Study the drawing (mm; zero at the part's minimum x, y, z) and answer. Give positions to 0.01 mm unless a question says otherwise; leave off trailing zeros. Order: outer loops, then holes, each group sorted by start corner. A loop starts at its lowest first (then second) coordinate and runs counter-clockwise, first axis right, second up. Notation, with made-up numbers: (39.5, 6.5) - (68.5, 6.5) arc R19 cw to (68.5, 14.5) - close; hole circle Ø11 at (89.25, 9.5). An arc over 180 degrees is marked (long way). Put each result on its own line as item: value.
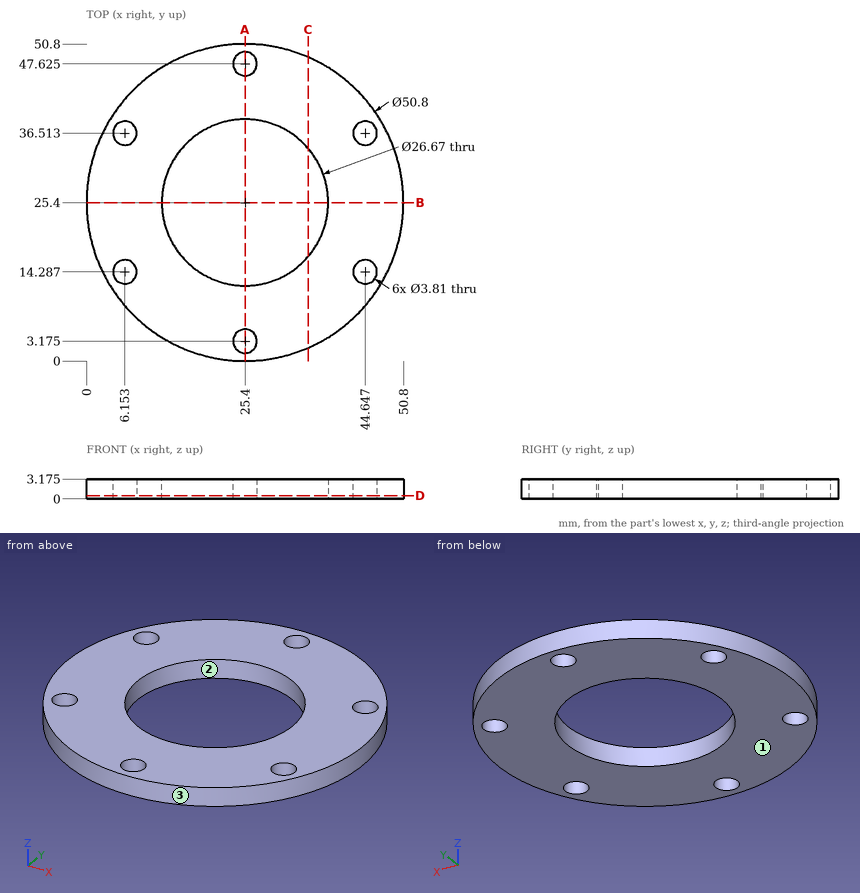
(1) Given pin 1 (1.5 mm diameter, centred on y = 22, z = 1, fed in from -X), flat-ended and moving along its own axis, determine where the tip first touches the part or whether it passes through.
Geometry check:
pin 1: stops at x = 0.14
(2) Section A-A, the plane x = 25.4 is taken. Write down the section's boundary in (y, z) (1 decimal).
Geometry check:
outline: (0, 0) - (1.3, 0) - (1.3, 3.2) - (0, 3.2) - close; (5.1, 0) - (12.1, 0) - (12.1, 3.2) - (5.1, 3.2) - close; (38.7, 0) - (45.7, 0) - (45.7, 3.2) - (38.7, 3.2) - close; (49.5, 0) - (50.8, 0) - (50.8, 3.2) - (49.5, 3.2) - close
(3) Section C-C, the plane x = 35.5 is taken. Write down the section's boundary in (y, z) (1 decimal).
Geometry check:
outline: (2.1, 0) - (16.7, 0) - (16.7, 3.2) - (2.1, 3.2) - close; (34.1, 0) - (48.7, 0) - (48.7, 3.2) - (34.1, 3.2) - close
(4) Determine the mould class of the marked faces 1, 2 and 3 for opening direction Y: pulls with the +Y half, pulls with the -Y half, needs draft (parallel to the pull), parting line crosses it, or undercut.
Geometry check:
face 1: needs draft
face 2: undercut
face 3: parting line crosses it
(5) Section D-D, the plane z = 0.5 is taken. Write down the section's boundary in (x, y) (1 decimal), then the cut area to 3 significant figures.
Geometry check:
outline: circle Ø50.8 at (25.4, 25.4); hole circle Ø3.8 at (6.2, 14.3); hole circle Ø3.8 at (6.2, 36.5); hole circle Ø26.7 at (25.4, 25.4); hole circle Ø3.8 at (25.4, 3.2); hole circle Ø3.8 at (25.4, 47.6); hole circle Ø3.8 at (44.6, 14.3); hole circle Ø3.8 at (44.6, 36.5)
area: 1,400 mm²
(6) Straight lines are drawn through the part: line 1 (Y direction, x = 25, z = 2.7); line 2 (Y direction, x = 24, z = 2) (1 decimal); line 3 (Y direction, x = 6, z = 1.45) (1 decimal). For each, find the intervals that lie inside material, in ascending order.
Geometry check:
line 1: y = 0 to 1.31, 5.04 to 12.07, 38.73 to 45.76, 49.49 to 50.8
line 2: y = 0 to 1.9, 4.5 to 12.1, 38.7 to 46.3, 48.9 to 50.8
line 3: y = 9 to 12.4, 16.2 to 34.6, 38.4 to 41.8
(7) Section B-B, the plane y = 25.4 is taken. Write down the section's boundary in (x, z) (1 decimal).
Geometry check:
outline: (0, 0) - (12.1, 0) - (12.1, 3.2) - (0, 3.2) - close; (38.7, 0) - (50.8, 0) - (50.8, 3.2) - (38.7, 3.2) - close
